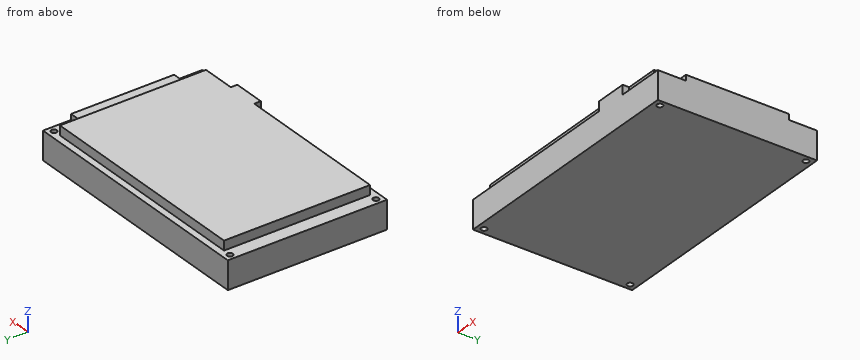
from build123d import *

# Parameters (mm, degrees)
F0_R     = 1.55
F1_DEPTH = 15
F2_W     = 17
F2_H     = 3.5
F3_DEPTH = 5
F4_W     = 7.5
F4_H     = 55
F5_DEPTH = 3


with BuildPart() as f1:
    # F0 (on Top) → F1 (new body)
    with BuildSketch(Plane.XY):
        with Locations((-3.25, 3.5)):
            Circle(F0_R)
        with BuildLine():
            ThreePointArc((-129.2, 81.5), (-130.75, 83.05), (-132.3, 81.5))
            ThreePointArc((-132.3, 81.5), (-130.75, 79.95), (-129.2, 81.5))
        make_face()
        with BuildLine():
            ThreePointArc((-129.2, 3.5), (-130.75, 5.05), (-132.3, 3.5))
            ThreePointArc((-132.3, 3.5), (-130.75, 1.95), (-129.2, 3.5))
        make_face()
        Polygon((-134, 0), (0, 0), (0, 3.5), (0, 81.5), (0, 85), (-134, 85), (-134, 81.5), (-134, 3.5), align=None)
        with BuildLine():
            ThreePointArc((-129.2, 3.5), (-130.75, 1.95), (-132.3, 3.5))
            ThreePointArc((-132.3, 3.5), (-130.75, 5.05), (-129.2, 3.5))
        make_face(mode=Mode.SUBTRACT)
        with Locations((-3.25, 3.5)):
            Circle(F0_R, mode=Mode.SUBTRACT)
        with BuildLine():
            ThreePointArc((-129.2, 81.5), (-130.75, 79.95), (-132.3, 81.5))
            ThreePointArc((-132.3, 81.5), (-130.75, 83.05), (-129.2, 81.5))
        make_face(mode=Mode.SUBTRACT)
        with BuildLine():
            ThreePointArc((-4.8, 81.5), (-3.25, 83.05), (-1.7, 81.5))
            ThreePointArc((-1.7, 81.5), (-3.25, 79.95), (-4.8, 81.5))
        make_face(mode=Mode.SUBTRACT)
    extrude(amount=F1_DEPTH)

    # F2 (on face) → F3 (join)
    with BuildSketch(Plane.XY.offset(15)):
        Polygon((-7.5, 3.5), (-7.5, 81.5), (-126.5, 81.5), (-126.5, 3.5), (-42.5, 3.5), (-25.5, 3.5), align=None)
        with Locations((-34, 1.75)):
            Rectangle(F2_W, F2_H)
    extrude(amount=F3_DEPTH)

    # F4 (on face) → F5 (join)
    with BuildSketch(Plane.XY.offset(15)):
        with Locations((-3.75, 42.5)):
            Rectangle(F4_W, F4_H)
    extrude(amount=F5_DEPTH)


solid = f1.part
Read the model definition and answer for the solid it produces. Units are mm, in the model's axes. Coordinates: 2 decimals unless noted, no trailing zeros. Loops run counter-clockwise (first coordinate to the right, second up) from the corner with the lowest first, then second, coordinate; pieces in that order, holes last.
Q1. The part is cut by section C-C on x = -116.5. Write down the section's boundary in (y, z), and give its area (4 significant figures).
Q2. Consider probe 1 along X at (y, z) = (81.5, 6.5); probe 2 along Y at (x, z) = (-3.25, 11); probe 3 along Z at (x, y) = (-6.5, 42.5). Determine where each line is inside the solid, lowest interval first.
Q3. The part is cut by section D-D on x = -130.75. Write down the section's boundary in (y, z).
Q4. The part is cut by section A-A on x = -3.25. Write down the section's boundary in (y, z).
Q5. The part is cut by section B-B on y = 56.5. Write down the section's boundary in (x, z), and give its area (3 significant figures).
Q6. Each of these flat-tipped pins is pushed along its axis until it touches: pin 1 Ø1 at (y, z) = (2, 17) entering from +X; pin 2 Ø8 at (x, y) = (-52.5, 25.5) entering from -Z; pin 3 Ø4 at (x, z) = (-39, 18.5) entering from +Y; pin 4 Ø0.9 at (x, z) = (-5, 17) entering from +Y. Where does it stop, or does it pass through?
Results below:
1. outline: (0, 0) - (85, 0) - (85, 15) - (81.5, 15) - (81.5, 20) - (3.5, 20) - (3.5, 15) - (0, 15) - close
1. area: 1,665 mm2
2. probe 1: x = -134 to -132.3, -129.2 to -4.8, -1.7 to 0
2. probe 2: y = 0 to 1.95, 5.05 to 79.95, 83.05 to 85
2. probe 3: z = 0 to 18
3. outline: (0, 0) - (1.95, 0) - (1.95, 15) - (0, 15) - close; (5.05, 0) - (79.95, 0) - (79.95, 15) - (5.05, 15) - close; (83.05, 0) - (85, 0) - (85, 15) - (83.05, 15) - close
4. outline: (0, 0) - (1.95, 0) - (1.95, 15) - (0, 15) - close; (5.05, 0) - (79.95, 0) - (79.95, 15) - (70, 15) - (70, 18) - (15, 18) - (15, 15) - (5.05, 15) - close; (83.05, 0) - (85, 0) - (85, 15) - (83.05, 15) - close
5. outline: (-134, 0) - (0, 0) - (0, 18) - (-7.5, 18) - (-7.5, 20) - (-126.5, 20) - (-126.5, 15) - (-134, 15) - close
5. area: 2,630 mm2
6. pin 1: stops at x = -25.5
6. pin 2: stops at z = 0
6. pin 3: stops at y = 81.5
6. pin 4: stops at y = 70
